Read the model definition and answer for the solid it produces. Units are mm, in the model's axes. Coordinates: 2 decimals unless noted, no trailing zeros.
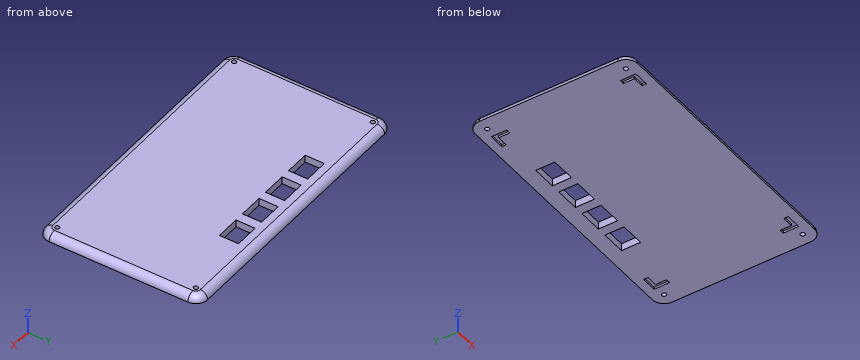
from build123d import *

# Parameters (mm, degrees)
F1_DEPTH = 5
F2_R     = 1.5
F3_DEPTH = 5.001
F4_DEPTH = 25
F5_R     = 4.99999
F6_W     = 16.5
F6_H     = 13
F7_DEPTH = 5.001
F9_DEPTH = 1.5


# Not quite as in the source:
# - a fillet or chamfer is up to 0.001 mm smaller than in the source, because OpenCascade refuses the exact size


with BuildPart() as f1:
    # F0 (on Top) → F1 (new body)
    with BuildSketch(Plane.XY):
        with BuildLine():
            ThreePointArc((-61.6726832837, -15.8819631437), (-59.3295375332, -21.5388173932), (-53.6726832837, -23.8819631437))
            Line((-53.6726832837, -23.8819631437), (122.8273167163, -23.8819631437))
            ThreePointArc((122.8273167163, -23.8819631437), (128.4841709658, -21.5388173932), (130.8273167163, -15.8819631437))
            Line((130.8273167163, -15.8819631437), (130.8273167163, 78.4180368563))
            ThreePointArc((130.8273167163, 78.4180368563), (128.4841709658, 84.0748911058), (122.8273167163, 86.4180368563))
            Line((122.8273167163, 86.4180368563), (-53.6726832837, 86.4180368563))
            ThreePointArc((-53.6726832837, 86.4180368563), (-59.3295375332, 84.0748911058), (-61.6726832837, 78.4180368563))
            Line((-61.6726832837, 78.4180368563), (-61.6726832837, -15.8819631437))
        make_face()
    extrude(amount=-F1_DEPTH)

    # F2 (on face) → F3 (cut, through all)
    with BuildSketch(Plane(origin=(0, 0, -5), x_dir=(1, 0, 0), z_dir=(0, 0, -1))):
        with Locations((-53.6726832837, 15.8819631437)):
            Circle(F2_R)
        with Locations((122.8273167163, 15.8819631437)):
            Circle(F2_R)
        with Locations((122.8273167163, -78.4180368563)):
            Circle(F2_R)
        with Locations((-53.6726832837, -78.4180368563)):
            Circle(F2_R)
    extrude(amount=-F3_DEPTH, mode=Mode.SUBTRACT)

    # F4 (cut): a face of the model
    f4_faces = [f1.faces().sort_by_distance(p)[0] for p in [
        (34.5773167163, 31.2680368563, -5),
    ]]
    extrude(f4_faces, amount=F4_DEPTH, mode=Mode.SUBTRACT)

    # F5 (radius 5 in the source; OpenCascade refuses exactly that, so slightly less here)
    f5_edges = [f1.edges().sort_by_distance(p)[0] for p in [
        (34.577317, 86.418037, 0),
        (128.484171, 84.074891, 0),
        (130.827317, 31.268037, 0),
        (128.484171, -21.538817, 0),
        (34.577317, -23.881963, 0),
        (-59.329538, -21.538817, 0),
        (-61.672683, 31.268037, 0),
        (-59.329538, 84.074891, 0),
    ]]
    fillet(f5_edges, radius=F5_R)

    # F6 (on face) → F7 (cut, through all)
    with BuildSketch(Plane.XY):
        with Locations((0.0773167163, 69.9180368563)):
            Rectangle(F6_W, F6_H)
        with Locations((23.0773167163, 69.9180368563)):
            Rectangle(F6_W, F6_H)
        with Locations((46.0773167163, 69.9180368563)):
            Rectangle(F6_W, F6_H)
        with Locations((69.0773167163, 69.9180368563)):
            Rectangle(F6_W, F6_H)
    extrude(amount=-F7_DEPTH, mode=Mode.SUBTRACT)

    # F8 (on face) → F9 (cut)
    with BuildSketch(Plane(origin=(0, 0, -5), x_dir=(1, 0, 0), z_dir=(0, 0, -1))):
        Polygon((-43.6726832837, -69.9180368563), (-46.6726832837, -69.9180368563), (-46.6726832837, -80.4180368563), (-36.1726832837, -80.4180368563), (-36.1726832837, -77.4180368563), (-43.6726832837, -77.4180368563), align=None)
        Polygon((-46.6726832837, 7.3819631437), (-43.6726832837, 7.3819631437), (-43.6726832837, 14.8819631437), (-36.1726832837, 14.8819631437), (-36.1726832837, 17.8819631437), (-46.6726832837, 17.8819631437), align=None)
        Polygon((115.8273167163, 17.8819631437), (105.3273167163, 17.8819631437), (105.3273167163, 14.8819631437), (112.8273167163, 14.8819631437), (112.8273167163, 7.3819631437), (115.8273167163, 7.3819631437), align=None)
        Polygon((115.8273167163, -69.9180368563), (112.8273167163, -69.9180368563), (112.8273167163, -77.4180368563), (105.3273167163, -77.4180368563), (105.3273167163, -80.4180368563), (115.8273167163, -80.4180368563), align=None)
    extrude(amount=-F9_DEPTH, mode=Mode.SUBTRACT)


solid = f1.part
Item 1: Given pin 1 (0.8 mm diameter, centred on y = 73.5, z = -4, fed in from -X); pin 2 (1.6 mm diameter, centred on x = 109, z = -4, fed in from +Y); pin 3 (1.5 mm diameter, centred on y = 71, z = -3.5, fed in from +X), each flat-ended and moving along its own axis, determine where each tip first touches the part or whether it passes through.
Numbers:
pin 1: stops at x = -61.64
pin 2: stops at y = 86.41
pin 3: stops at x = 130.77
Item 2: Find the intervals of material crossed by line 1 along X through (y, z) = (21.5, -4.45); line 2 along X through (y, z) = (78.5, -1.95); line 3 along Y through (x, z) = (117.5, -4.6), in increasing order.
Numbers:
line 1: x = -61.64 to 130.8
line 2: x = -60.63 to -55.17, -52.17 to 121.33, 124.33 to 129.79
line 3: y = -23.87 to 86.4
Item 3: A cutting plane is placed at A-A on y = 73.5. Give the number of separate pieces and of enclosed holes in the cut face, then the cut area to 3 significant figures.
Numbers:
separate pieces: 5
enclosed holes: 0
area: 613 mm2
